```python
from build123d import *

# Parameters (mm, degrees)
F0_W     = 60
F0_H     = 60
F1_DEPTH = 6
F2_W     = 47
F2_H     = 47
F3_DEPTH = 3
F4_W     = 47
F4_H     = 4
F5_DEPTH = 20
F6_W     = 25
F6_H     = 30
F7_DEPTH = 25


with BuildPart() as f1:
    # F0 (on Top) → F1 (new body)
    with BuildSketch(Plane.XY):
        with Locations((30, 90)):
            Rectangle(F0_W, F0_H)
        with Locations((30, 30)):
            Rectangle(F0_W, F0_H)
    extrude(amount=F1_DEPTH)

    # F2 (on face) → F3 (cut)
    with BuildSketch(Plane.XY.offset(6)):
        with Locations((30.5, 89.5)):
            Rectangle(F2_W, F2_H)
        with Locations((30.5, 30.5)):
            Rectangle(F2_W, F2_H)
    extrude(amount=-F3_DEPTH, mode=Mode.SUBTRACT)

    # F4 (on Top) → F5 (join)
    with BuildSketch(Plane.XY):
        with Locations((30.5, 60)):
            Rectangle(F4_W, F4_H)
    extrude(amount=F5_DEPTH)

    # F6 (on Top) → F7 (cut)
    with BuildSketch(Plane.XY):
        with Locations((30.5, 30)):
            Rectangle(F6_W, F6_H)
        with Locations((30.5, 90)):
            Rectangle(F6_W, F6_H)
    extrude(amount=F7_DEPTH, mode=Mode.SUBTRACT)


solid = f1.part
```
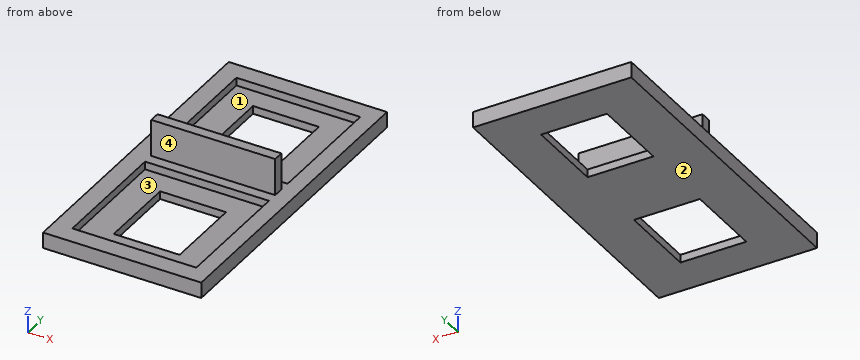
Can you work these out from the model? Positions are in its coordinate system, mm. Face numbers are marked on the shaded views. Give positions to 0.01 mm unless a question says otherwise; leave off trailing zeros. Loops run counter-clockwise (first coordinate to the right, second up) from the corner with the lowest first, then second, coordinate; pieces in that order, holes last. Notation, with made-up numbers: M 14.25,68.25 L 58.25,68.25 A26 ccw 58.25,93.25 Z; hole C 79,78.25 d10. An arc over 180 degrees is marked long. Answer in a Markdown table with one row per item.
1. Suppose I cut it at D-D on y = 67.5. Write out the boundary of the cut face in (x, z), plus the area to 3 significant figures.
Taken from the geometry:
| item | result |
|---|---|
| outline | M 0,0 L 60,0 L 60,6 L 54,6 L 54,3 L 7,3 L 7,6 L 0,6 Z |
| area | 219 mm² |
2. Suppose I cut it at C-C on x = 36. Write out the boundary of the cut face in (y, z).
Taken from the geometry:
| item | result |
|---|---|
| outline | M 0,0 L 15,0 L 15,3 L 7,3 L 7,6 L 0,6 Z; M 45,0 L 75,0 L 75,3 L 66,3 L 66,6 L 62,6 L 62,20 L 58,20 L 58,6 L 54,6 L 54,3 L 45,3 Z; M 105,0 L 120,0 L 120,6 L 113,6 L 113,3 L 105,3 Z |
3. Suppose I cut it at B-B on z = 4.5. Write out the boundary of the cut face in (x, y).
Taken from the geometry:
| item | result |
|---|---|
| outline | M 0,0 L 60,0 L 60,120 L 0,120 Z; hole M 7,7 L 54,7 L 54,54 L 7,54 Z; hole M 7,66 L 54,66 L 54,113 L 7,113 Z |
4. Thinking about a two-plate mould opening in Y: for the marked faces 1, 2, 3 and 4, which applies, released by +Y, released by -Y, zero draft, split by the parting line, or undercut?
Taken from the geometry:
| item | result |
|---|---|
| face 1 | undercut |
| face 2 | zero draft |
| face 3 | undercut |
| face 4 | released by -Y |
5. Suppose I cut it at A-A on y = 20.5. Write out the boundary of the cut face in (x, z).
Taken from the geometry:
| item | result |
|---|---|
| outline | M 0,0 L 18,0 L 18,3 L 7,3 L 7,6 L 0,6 Z; M 43,0 L 60,0 L 60,6 L 54,6 L 54,3 L 43,3 Z |
6. For pin 1 Ø5 at (x, z) = (25.5, 14) entering from -Y; pin 2 Ø10 at (y, z) = (16.5, 13) entering from -X; pin 3 Ø6 at (x, y) = (20.5, 15) entering from +Z; pin 4 Ø3 at (y, z) = (60, 11) entering from -X, each with a flat end and sliding along its axis, tell me the tip position at first contact or that it passes through.
Taken from the geometry:
| item | result |
|---|---|
| pin 1 | stops at y = 58 |
| pin 2 | passes through |
| pin 3 | stops at z = 3 |
| pin 4 | stops at x = 7 |
7. If I drill on line 1 along Y through (x, z) = (33, 3.25); line 2 along Y through (x, z) = (27, 2.25); line 3 along X through (y, z) = (78.5, 5.5), over which ranges is the centre line in solid material (lowest first)?
Taken from the geometry:
| item | result |
|---|---|
| line 1 | y = 0 to 7, 54 to 66, 113 to 120 |
| line 2 | y = 0 to 15, 45 to 75, 105 to 120 |
| line 3 | x = 0 to 7, 54 to 60 |
